Study the drawing (mm; zero at the part's minimum x, y, z) and answer. A direction names the side the tool comes from. Coordinates: 2 decimals unless noted, no trailing zeros. Write each loop counter-clockwise with the first axis right and the second up, starting at its lowest first coordinate (ties: lowest second). Pieces come first, ordered by that corner, then holes. Notation, with made-up numbers: (44.25, 53) - (71.25, 53) arc R28 cw to (71.25, 90) - close; hole circle Ø11 at (26, 77.5). An arc over 180 degrees is marked (long way). One line per item, written item: value.
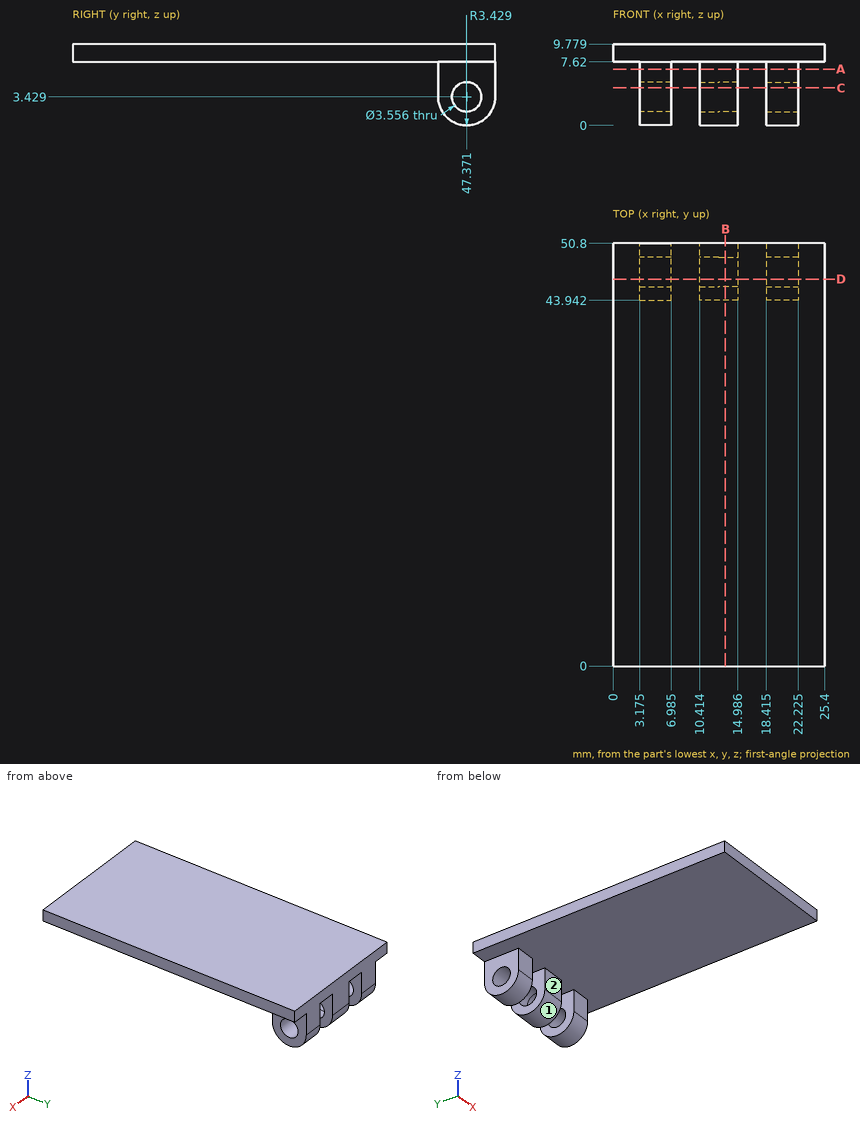
Item 1: Which of the six approach directions +Z, -Z, +X, -X, +Y, -Y give full straight-line access (tool end or side, diameter ignored) to the marked faces 1 and 2?
Evaluation:
face 1: -Z, +X, -X
face 2: -Z, +X, -X, -Y
Item 2: Given pin 1 (4 mm diameter, centred on y = 47.371, z = 3.429, fed in from +X) (3 decimals); pin 2 (5 mm diameter, centred on x = 22.5, z = 6, fed in from -Y); pin 3 (2 mm diameter, centred on x = 23, z = 6.5, fed in from -Y); pin 4 (12.5 mm diameter, centred on x = 18.5, y = 34, fed in from -Z), each flat-ended and moving along its own axis, determine where each tip first touches the part or whether it passes through.
Evaluation:
pin 1: stops at x = 22.225
pin 2: stops at y = 0
pin 3: stops at y = 43.94
pin 4: stops at z = 7.62
Item 3: Section A-A, the plane z = 6.75 is taken. Determine the outline of the cut face in (x, y) (3 decimals).
Evaluation:
outline: (3.175, 43.942) - (6.985, 43.942) - (6.985, 50.8) - (3.175, 50.8) - close; (10.414, 43.942) - (14.986, 43.942) - (14.986, 50.8) - (10.414, 50.8) - close; (18.415, 43.942) - (22.225, 43.942) - (22.225, 50.8) - (18.415, 50.8) - close
Item 4: Section C-C, the plane z = 4.5 is taken. Determine the outline of the cut face in (x, y) (3 decimals), then the cut area to 3 significant figures.
Evaluation:
outline: (3.175, 43.942) - (6.985, 43.942) - (6.985, 45.952) - (3.175, 45.952) - close; (3.175, 48.79) - (6.985, 48.79) - (6.985, 50.8) - (3.175, 50.8) - close; (10.414, 43.942) - (14.986, 43.942) - (14.986, 45.952) - (10.414, 45.952) - close; (10.414, 48.79) - (14.986, 48.79) - (14.986, 50.8) - (10.414, 50.8) - close; (18.415, 43.942) - (22.225, 43.942) - (22.225, 45.952) - (18.415, 45.952) - close; (18.415, 48.79) - (22.225, 48.79) - (22.225, 50.8) - (18.415, 50.8) - close
area: 49.0 mm2
Item 5: Consider probe 1 along Z at (x, y) = (15.25, 20); probe 2 along Y at (x, z) = (19.25, 5); probe 3 along Y at (x, z) = (19, 6.5). Determine where each line is inside the solid, lowest interval first.
Evaluation:
probe 1: z = 7.62 to 9.78
probe 2: y = 43.94 to 46.54, 48.2 to 50.8
probe 3: y = 43.94 to 50.8
Item 6: Section B-B, the plane x = 13.5 is taken. Determine the outline of the cut face in (y, z).
Evaluation:
outline: (0, 7.62) - (43.94, 7.62) - (43.94, 3.43) arc R3.43 ccw to (50.8, 3.43) - (50.8, 9.78) - (0, 9.78) - close; hole circle Ø3.56 at (47.37, 3.43)
Item 7: Section D-D, the plane y = 46.5 is taken. Determine the outline of the cut face in (x, z) (3 decimals).
Evaluation:
outline: (0, 7.62) - (3.175, 7.62) - (3.175, 4.979) - (6.985, 4.979) - (6.985, 7.62) - (10.414, 7.62) - (10.414, 4.979) - (14.986, 4.979) - (14.986, 7.62) - (18.415, 7.62) - (18.415, 4.979) - (22.225, 4.979) - (22.225, 7.62) - (25.4, 7.62) - (25.4, 9.779) - (0, 9.779) - close; (3.175, 0.112) - (6.985, 0.112) - (6.985, 1.879) - (3.175, 1.879) - close; (10.414, 0.112) - (14.986, 0.112) - (14.986, 1.879) - (10.414, 1.879) - close; (18.415, 0.112) - (22.225, 0.112) - (22.225, 1.879) - (18.415, 1.879) - close
